Geometry check sheet. Reference: the model listing, model coordinates, mm. A direction names the side the tool comes from. Round coordinates to 2 decimals unless told otherwise and drop trailing zeros. Loops run counter-clockwise (first coordinate to the right, second up) from the corner with the lowest first, then second, coordinate; pieces in that order, holes last. Notation, with made-up numbers: (89, 16.25) -> (109, 16.25) arc R12 cw to (109, 29.25) -> close; hole circle Ø9 at (-18, -36.75). An arc over 180 degrees is marked (long way). Use a Markdown table: item, result. Add a question column.
Q1. Gauge pin test, flat ends, axial feed: P1, Ø4, axis at y = 7.5, z = 46.5, coming from the -X side; P2, Ø18.5, axis at x = 38.1, y = 12.7, coming from the +Z side; P3, Ø2, axis at y = 23, z = 1, coming from the +X side; P4, Ø6, axis at y = 12, z = 29, coming from the -X side. Record the tip position at first contact, or that the pin passes through.
Q2. Material ranges on L1, parallel to Y at x = 38, z = 44; L2, parallel to Z at x = 43.5, y = 25; L3, parallel to Y at x = 18, z = -3, recorded low to high.
Q3. Sectioned sample at A-A, the plane y = 12.7. Enter the section's corners in (x, z).
Q4. Release check for a two-part mould opening along Y. For faces 1 (the face through (-49.014, 18.783, 48.224)), 2 (the face through (28.41, 15.75, -50.62)), 3 (the face through (-15, 0, -1)) record: released by +Y, released by -Y, zero draft, split by the parting line, or undercut.
Q5. Sectioned sample at D-D, the plane z = -3. Enter the section's corners in (x, y), then the cut area to 3 significant figures.
Q6. Sectioned sample at B-B, the plane x = 38.1. Give the number of separate pieces and of enclosed holes in the cut face, then the cut area to 3 significant figures.
Q7. Set-up check for faces 4 (the face through (28.41, 15.75, 50.98)), 5 (the face through (44, 4, -38.1)): record each of +Z, -Z, +X, -X, +Y, -Y from which the full face is reachable in a straight line by a thin tool's end or side.
```python
from build123d import *

# Parameters (mm, degrees)
BOSS_EXTRUDE1_DEPTH     = 38.1
SKETCH2_W               = 76.2
SKETCH2_H               = 50.8
CUT_EXTRUDE1_DEPTH      = 50.8
CUT_EXTRUDE2_DEPTH      = 126.723585695
CUT_EXTRUDE2_DEPTH_BACK = 126.723585695
SKETCH3_R               = 10.16
SKETCH6_W               = 76.223232364
SKETCH6_H               = 12.7
CUT_EXTRUDE4_DEPTH      = 38.1


with BuildPart() as part:
    # Sketch1 → Boss-Extrude1 (new body)
    with BuildSketch(Plane(origin=(0, 0, 0), x_dir=(1, 0, 0), z_dir=(0, 1, 0))):
        with BuildLine():
            Line((63.5, 63.5), (-12.7, 63.5))
            ThreePointArc((-12.7, 63.5), (-48.621024484, 48.621024484), (-63.5, 12.7))
            Line((-63.5, 12.7), (-63.5, -12.7))
            ThreePointArc((-63.5, -12.7), (-48.621024484, -48.621024484), (-12.7, -63.5))
            Line((-12.7, -63.5), (63.5, -63.5))
            Line((63.5, -63.5), (63.5, 63.5))
        make_face()
    extrude(amount=BOSS_EXTRUDE1_DEPTH)

    # Sketch2 → Cut-Extrude1 (cut)
    with BuildSketch(Plane(origin=(63.5, 0, 0), x_dir=(0, 0, -1), z_dir=(1, 0, 0))):
        Rectangle(SKETCH2_W, SKETCH2_H)
    extrude(amount=-CUT_EXTRUDE1_DEPTH, mode=Mode.SUBTRACT)

    # Sketch3 → Cut-Extrude2 (cut, two sides: drawn at the far end of the back side and taken through both)
    with BuildSketch(Plane(origin=(0, 0, 38.1), x_dir=(-1, 0, 0), z_dir=(0, 0, -1)).offset(-CUT_EXTRUDE2_DEPTH_BACK)):
        with Locations((-38.1, 12.7)):
            Circle(SKETCH3_R)
    extrude(amount=CUT_EXTRUDE2_DEPTH + CUT_EXTRUDE2_DEPTH_BACK, mode=Mode.SUBTRACT)

    # Sketch6 → Cut-Extrude4 (cut)
    with BuildSketch(Plane(origin=(63.5, 0, 0), x_dir=(0, 0, -1), z_dir=(1, 0, 0))):
        with Locations((0.011616182, 31.75)):
            Rectangle(SKETCH6_W, SKETCH6_H)
    extrude(amount=-CUT_EXTRUDE4_DEPTH, mode=Mode.SUBTRACT)


solid = part.part
```
Values:
| question | item | result |
|---|---|---|
| 1 | P1 | x = -52.32 |
| 1 | P2 | through |
| 1 | P3 | x = 12.7 |
| 1 | P4 | x = -61.73 |
| 2 | L1 | 0 to 2.54, 22.86 to 38.1 |
| 2 | L2 | -63.5 to -38.1, 38.1 to 63.5 |
| 2 | L3 | 25.4 to 38.1 |
| 3 | outline | (-63.5, -12.7) arc R50.8 ccw to (-12.7, -63.5) -> (27.94, -63.5) -> (27.94, -38.1) -> (12.7, -38.1) -> (12.7, 38.1) -> (27.94, 38.1) -> (27.94, 63.5) -> (-12.7, 63.5) arc R50.8 ccw to (-63.5, 12.7) -> close; (48.26, -63.5) -> (63.5, -63.5) -> (63.5, -38.1) -> (48.26, -38.1) -> close; (48.26, 38.1) -> (63.5, 38.1) -> (63.5, 63.5) -> (48.26, 63.5) -> close |
| 4 | face 1 | zero draft |
| 4 | face 2 | undercut |
| 4 | face 3 | released by -Y |
| 5 | outline | (-63.5, 0) -> (12.7, 0) -> (12.7, 25.4) -> (25.4, 25.4) -> (25.4, 38.1) -> (-63.5, 38.1) -> close |
| 5 | area | 3,060 mm^2 |
| 6 | separate pieces | 4 |
| 6 | enclosed holes | 0 |
| 6 | area | 903 mm^2 |
| 7 | face 4 | +Z, -Z |
| 7 | face 5 | +X, -Y |
